```python
from build123d import *

# Parameters (mm, degrees)
SKETCH1_R           = 1.75
SKETCH1_R_2         = 2.4
BOSS_EXTRUDE1_DEPTH = 4
CUT_EXTRUDE1_DEPTH  = 10


with BuildPart() as part:
    # Sketch1 → Boss-Extrude1 (new body)
    with BuildSketch(Plane(origin=(-201.849311144, 125.418002604, 0.593848714), x_dir=(0.5277644625295516, 0.8493907652493602, 0), z_dir=(0.8493881131629323, -0.5277628146696672, -0.002498933665448049))):
        with BuildLine():
            Line((162.208427101, 97.881301323), (161.820912094, 98.53237983))
            ThreePointArc((161.820912094, 98.53237983), (162.176155218, 98.906966779), (162.515086857, 99.296374539))
            ThreePointArc((162.515086857, 99.296374539), (163.723385062, 98.699566989), (165.041833408, 98.420536953))
            ThreePointArc((165.041833408, 98.420536953), (165.22305653, 98.674638573), (165.398816038, 98.932549505))
            ThreePointArc((165.398816038, 98.932549505), (164.681084034, 100.073174148), (163.703268012, 101.000557365))
            ThreePointArc((163.703268012, 101.000557365), (161.330105787, 116.014599459), (146.152484133, 116.847161686))
            Line((146.152484133, 116.847161686), (130.289477893, 127.907081314))
            ThreePointArc((130.289477893, 127.907081314), (124.720550757, 126.913577135), (125.714054936, 121.344649999))
            Line((125.714054936, 121.344649999), (141.577061176, 110.284730371))
            ThreePointArc((141.577061176, 110.284730371), (141.428783224, 109.695705854), (141.310268829, 109.099978927))
            ThreePointArc((141.310268829, 109.099978927), (139.965448113, 109.012680325), (138.684123333, 108.595103251))
            ThreePointArc((138.684123333, 108.595103251), (138.654230316, 108.284433232), (138.630973584, 107.973196059))
            ThreePointArc((138.630973584, 107.973196059), (139.822860053, 107.344252144), (141.133365177, 107.03002273))
            ThreePointArc((141.133365177, 107.03002273), (141.145956651, 106.487309655), (141.182892388, 105.945708529))
            ThreePointArc((141.182892388, 105.945708529), (139.906489868, 105.513319341), (138.776902071, 104.778339605))
            ThreePointArc((138.776902071, 104.778339605), (138.828434951, 104.470518528), (138.88652478, 104.163867219))
            ThreePointArc((138.88652478, 104.163867219), (140.200581367, 103.864836966), (141.547760668, 103.900498345))
            ThreePointArc((141.547760668, 103.900498345), (141.700387578, 103.379536682), (141.876241447, 102.86594984))
            ThreePointArc((141.876241447, 102.86594984), (140.755241845, 102.117936675), (139.854370572, 101.115641931))
            ThreePointArc((139.854370572, 101.115641931), (139.983817469, 100.831647293), (140.119295134, 100.550479629))
            ThreePointArc((140.119295134, 100.550479629), (141.465971053, 100.601741456), (142.758016489, 100.984863363))
            ThreePointArc((142.758016489, 100.984863363), (143.040277563, 100.521155789), (143.343065412, 100.070583325))
            ThreePointArc((143.343065412, 100.070583325), (142.453862998, 99.057922043), (141.843101138, 97.856617022))
            ThreePointArc((141.843101138, 97.856617022), (142.04164046, 97.61580259), (142.245273383, 97.379279681))
            ThreePointArc((142.245273383, 97.379279681), (143.532794895, 97.777340179), (144.681655704, 98.481813489))
            ThreePointArc((144.681655704, 98.481813489), (145.074315316, 98.10696091), (145.483402655, 97.750108592))
            ThreePointArc((145.483402655, 97.750108592), (144.886595105, 96.541810387), (144.607565069, 95.22336204))
            ThreePointArc((144.607565069, 95.22336204), (144.861666689, 95.042138918), (145.119577621, 94.866379411))
            ThreePointArc((145.119577621, 94.866379411), (146.260202264, 95.584111414), (147.18758548, 96.561927437))
            ThreePointArc((147.18758548, 96.561927437), (147.663884528, 96.301475435), (148.15139273, 96.062662159))
            ThreePointArc((148.15139273, 96.062662159), (147.887651491, 94.741070557), (147.959368715, 93.395328961))
            ThreePointArc((147.959368715, 93.395328961), (148.251716028, 93.286047206), (148.546328766, 93.183028819))
            ThreePointArc((148.546328766, 93.183028819), (149.462324855, 94.171520079), (150.105030845, 95.356042267))
            ThreePointArc((150.105030845, 95.356042267), (150.632510335, 95.227740216), (151.165216521, 95.123240713))
            ThreePointArc((151.165216521, 95.123240713), (151.252515124, 93.778419997), (151.670092198, 92.497095217))
            ThreePointArc((151.670092198, 92.497095217), (151.980762217, 92.4672022), (152.29199939, 92.443945468))
            ThreePointArc((152.29199939, 92.443945468), (152.920943305, 93.635831937), (153.235172718, 94.946337061))
            ThreePointArc((153.235172718, 94.946337061), (153.777885794, 94.958928535), (154.319486919, 94.995864272))
            ThreePointArc((154.319486919, 94.995864272), (154.751876108, 93.719461752), (155.486855844, 92.589873955))
            ThreePointArc((155.486855844, 92.589873955), (155.794676921, 92.641406835), (156.10132823, 92.699496665))
            ThreePointArc((156.10132823, 92.699496665), (156.400358482, 94.013553251), (156.364697104, 95.360732552))
            ThreePointArc((156.364697104, 95.360732552), (156.885658766, 95.513359462), (157.399245608, 95.689213331))
            ThreePointArc((157.399245608, 95.689213331), (158.147258774, 94.568213729), (159.149553518, 93.667342456))
            ThreePointArc((159.149553518, 93.667342456), (159.433548155, 93.796789353), (159.71471582, 93.932267018))
            ThreePointArc((159.71471582, 93.932267018), (159.663453993, 95.278942937), (159.280332086, 96.570988373))
            ThreePointArc((159.280332086, 96.570988373), (159.744039659, 96.853249447), (160.194612124, 97.156037296))
            ThreePointArc((160.194612124, 97.156037296), (161.207273405, 96.266834883), (162.408578427, 95.656073022))
            ThreePointArc((162.408578427, 95.656073022), (162.649392859, 95.854612345), (162.885915768, 96.058245267))
            ThreePointArc((162.885915768, 96.058245267), (162.629922136, 97.000525318), (162.208427101, 97.881301323))
        make_face()
        with Locations(Location((128.001766415, 124.625865657, 0), (0, 0, 180))):
            Circle(SKETCH1_R, mode=Mode.SUBTRACT)
        with Locations(Location((153.226111782, 107.039083666, 0), (0, 0, 180))):
            Circle(SKETCH1_R_2, mode=Mode.SUBTRACT)
    extrude(amount=-BOSS_EXTRUDE1_DEPTH)

    # Sketch3 → Cut-Extrude1 (cut)
    with BuildSketch(Plane(origin=(-201.849311144, 125.418002604, 0.593848714), x_dir=(-0.0021225711784023066, 0.0013188483828421916, -0.9999968776603934), z_dir=(0.8493881131629325, -0.527762814669667, -0.002498933665448049))):
        with BuildLine():
            Line((-111.455565577, 150.432166351), (-103.598152949, 157.159486839))
            ThreePointArc((-103.598152949, 157.159486839), (-102.54066254, 157.077547623), (-102.622601756, 156.020057214))
            Line((-102.622601756, 156.020057214), (-110.480014384, 149.292736726))
            ThreePointArc((-110.480014384, 149.292736726), (-111.537504793, 149.374675942), (-111.455565577, 150.432166351))
        make_face()
    extrude(amount=-CUT_EXTRUDE1_DEPTH, mode=Mode.SUBTRACT)


solid = part.part
```
Input: part model. Units: mm. Frame: model coordinates. A direction names the side the tool comes from. Round coordinates to 2 decimals unless told otherwise and drop trailing zeros. Write each loop counter-clockwise with the first axis right and the second up, starting at its lowest first coordinate (ties: lowest second). Pieces come first, ordered by that corner, then holes. Notation, with made-up numbers: (62, 11) - (96, 11) arc R26 ccw to (96, 48) - close; hole circle Ø5 at (40, 23). An arc over 180 degrees is marked (long way). Write item = value, one per line.
(1) Access query for faces 1 (the cylindrical face through (-119.01, 262.01, 97.45)), 2 (the cylindrical face through (-128.126, 247.336, 99.672)), 3 (the cylindrical face through (-124.449, 253.277, 94.755)). Directions: +Z, -Z, +X, -X, +Y, -Y. A direction counts if a zero-diameter tool reaches every point of the face in a straight line with its end or side. Return the directions, or none.
Geometry check:
face_1 = none
face_2 = -X, -Y
face_3 = -Z
(2) Pull-direction query (Y, two-part tool) for faces 4 (the cylindrical face through (-118.249, 263.246, 96.876)), 5 (the cylindrical face through (-121.11, 258.66, 93.24)), 6 (the cylindrical face through (-129.512, 245.066, 107.949)); classes: +Y half, -Y half, draft (parallel to the pull), parting line (faces both ways), or undercut.
Geometry check:
face_4 = undercut
face_5 = +Y half
face_6 = -Y half
(3) Material intervals for probe 1 along Y at (x, z) = (-124.75, 96.5); probe 2 along Y at (x, z) = (-126.25, 115.5); probe 3 along X at (y, z) = (262.5, 96), sorted ascending.
Geometry check:
probe_1 = 249.05 to 250.13, 251.87 to 256.63
probe_2 = 246.54 to 254.12
probe_3 = -121.1 to -119.98
(4) Section query A-A on y = 241. Output: boundary loops of the cut face in (x, z).
Geometry check:
outline = (-134.4, 116.33) - (-129.7, 114.59) - (-129.67, 124.33) - (-134.37, 126.07) - close
(5) Contact query for flat-ended pins moving along their axis: pin 1 Ø4 at (x, z) = (-127.5, 100) entering from -Y; pin 2 Ø2 at (x, y) = (-128.5, 244.5) entering from +Z; pin 3 Ø10 at (x, y) = (-118.5, 250.5) entering from +Z. Output: stop coordinate, or through.
Geometry check:
pin_1 = 244.08
pin_2 = 122.53
pin_3 = 119.7
